Check sheet for the modelled part. Datum: model origin and axes. Units: mm. Round coordinates to 2 decimals unless told otherwise and drop trailing zeros. Loops run counter-clockwise (first coordinate to the right, second up) from the corner with the lowest first, then second, coordinate; pieces in that order, holes last. Notation, with made-up numbers: (19.25, 56.5) - (60.25, 56.5) arc R8 ccw to (60.25, 62.5) - close; hole circle Ø2 at (-15, 84.5). An arc over 180 degrees is marked (long way). Put each result on its own line as item: value.
Autodesk Inventor part; units mm, degrees
ref_plane "YZ Plane" through (0, 0, 0) normal (1, 0, 0) x (0, 1, 0)
ref_plane "XZ Plane" through (0, 0, 0) normal (0, 1, 0) x (-1, 0, 0)
ref_plane "XY Plane" through (0, 0, 0) normal (0, 0, 1) x (1, 0, 0)
sketch "Sketch1" plane through (0, 0, 0) normal (0, 0, 1) x (1, 0, 0)
  circle A0 centre (0, 0) radius 8
  dimension "d0" = 16
extrude "Extrusion1" add sketch "Sketch1" along normal blind 5
sketch "Sketch2" plane through (0, 0, 5) normal (0, 0, 1) x (1, 0, 0)
  circle A0 centre (0, 0) radius 8
  circle A1 centre (0, 0) radius 3.75
  dimension "d3" = 7.5
extrude "Extrusion2" cut sketch "Sketch2" against normal blind 5 contours A1
chamfer "Chamfer1" distance 1 angle 45 1 edges at (-3.75, 0, 5)
chamfer "Chamfer2" distance 1 angle 45 1 edges at (-8, 0, 5)
properties part number "SpoolHandle-stop1"
Item 1: Section check A-A on x = 0. Enter the section's corners in (y, z), then the cut area to 3 significant figures.
Filled sheet:
outline: (-8, 0) - (-3.75, 0) - (-3.75, 4) - (-4.75, 5) - (-7, 5) - (-8, 4) - close; (3.75, 0) - (8, 0) - (8, 4) - (7, 5) - (4.75, 5) - (3.75, 4) - close
area: 40.5 mm²
Item 2: Thickness scan on line 1 (Y direction, x = 0, z = 3); line 2 (Y direction, x = 2, z = 0.55); line 3 (X direction, y = -0.25, z = 0.8). Record the ranges inside material, lowest first. Write a range as from..to.
Filled sheet:
line 1: -8..-3.75, 3.75..8
line 2: -7.75..-3.17, 3.17..7.75
line 3: -8..-3.74, 3.74..8
Item 3: Release check for a two-part mould opening along X. For faces 1 (the flat face through (1, -5, 5)), 2 (the cylindrical face through (-1.73, 7.81, 1.97)), 3 (the cylindrical face through (-3.746, 0.165, 2.028)) record: +X half, -X half, draft (parallel to the pull), parting line (faces both ways), or undercut.
Filled sheet:
face 1: draft
face 2: parting line
face 3: undercut
Item 4: Section check C-C on z = 2.2. Enter the section's corners in (x, y).
Filled sheet:
outline: circle Ø16 at (0, 0); hole circle Ø7.5 at (0, 0)
Item 5: Go/stop test with flat-tipped pins: pin 1 (3 mm diameter, centred on y = 2.5, z = 2.5, fed in from -X); pin 2 (1.5 mm diameter, centred on y = 5.5, z = 3.5, fed in from -X); pin 3 (2 mm diameter, centred on x = 6, z = 3, fed in from -Y) (3 decimals). Record where each tip stops, or that it passes through.
Filled sheet:
pin 1: x = -7.94
pin 2: x = -6.44
pin 3: y = -6.245
